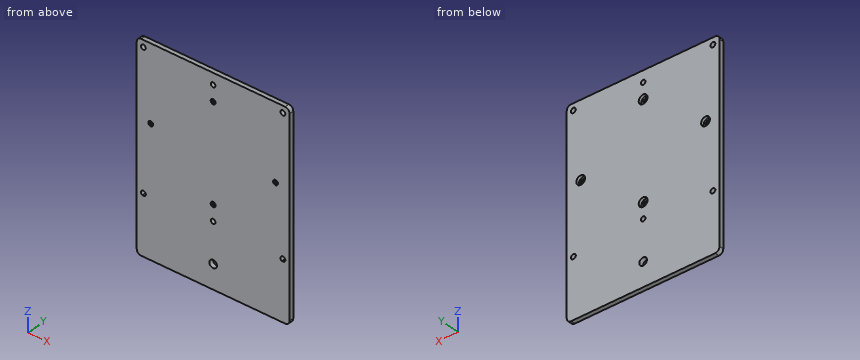
from build123d import *

# Parameters (mm, degrees)
SKETCH_1_W                   = 104
SKETCH_1_H                   = 100
EXTRUDE_1_DEPTH              = 3
HOLE_WIZARD_3_3_3_3_1_D      = 3.3
HOLE_WIZARD_M3_1_D           = 3.3
HOLE_WIZARD_M3_1_CBORE_D     = 6
HOLE_WIZARD_M3_1_CBORE_DEPTH = 2
FILLET_1_R                   = 3
SKETCH_49_R                  = 1.55
CUT_EXTRUDE_44_DEPTH         = 145.308696897
SKETCH_50_W                  = 104
SKETCH_50_H                  = 38
EXTRUDE_2_DEPTH              = 3
SKETCH_51_R                  = 2.6
CUT_EXTRUDE_45_DEPTH         = 145.308696897
FILLET_2_R                   = 3


with BuildPart() as part:
    # 草图1 → 凸台-拉伸1 (new body)
    with BuildSketch(Plane.XZ):
        with Locations((52, 50)):
            Rectangle(SKETCH_1_W, SKETCH_1_H)
    extrude(amount=-EXTRUDE_1_DEPTH)

    # Ø3.3 (3.3) 直径孔1 (through all)
    with Locations(Plane(origin=(0, 0, 0), x_dir=(-1, 0, 0), z_dir=(0, -1, 0))):
        with Locations((-4.5, -4.5), (-99.5, -4.5), (-99.5, -95.5), (-4.5, -95.5)):
            Hole(HOLE_WIZARD_3_3_3_3_1_D / 2)

    # M3 六角头机械螺钉的柱形沉头孔1 (through all)
    with Locations(Plane(origin=(0, 3, 0), x_dir=(1, 0, 0), z_dir=(0, 1, 0))):
        with Locations((52, -18), (94.5, -50), (9.5, -50), (52, -82)):
            CounterBoreHole(HOLE_WIZARD_M3_1_D / 2, HOLE_WIZARD_M3_1_CBORE_D / 2, HOLE_WIZARD_M3_1_CBORE_DEPTH)

    # 圆角1
    fillet_1_edges = [part.edges().sort_by_distance(p)[0] for p in [
        (0, 1.5, 100),
        (104, 1.5, 100),
        (104, 1.5, 0),
        (0, 1.5, 0),
    ]]
    fillet(fillet_1_edges, radius=FILLET_1_R)

    # 草图49 → 切除-拉伸44 (cut, through all)
    with BuildSketch(Plane(origin=(0, 3, 0), x_dir=(1, 0, 0), z_dir=(0, 1, 0))):
        with Locations(Location((52, -7.5, 0), (0, 0, 270))):
            Circle(SKETCH_49_R)
        with Locations(Location((52, -92.5, 0), (0, 0, 90))):
            Circle(SKETCH_49_R)
    extrude(amount=-CUT_EXTRUDE_44_DEPTH, mode=Mode.SUBTRACT)

    # 草图50 → 凸台-拉伸2 (add)
    with BuildSketch(Plane(origin=(0, 3, 0), x_dir=(1, 0, 0), z_dir=(0, 1, 0))):
        with Locations((52, 16)):
            Rectangle(SKETCH_50_W, SKETCH_50_H)
    extrude(amount=-EXTRUDE_2_DEPTH)

    # 草图51 → 切除-拉伸45 (cut, through all)
    with BuildSketch(Plane(origin=(0, 3, 0), x_dir=(1, 0, 0), z_dir=(0, 1, 0))):
        with Locations(Location((52, 19, 0), (0, 0, 270))):
            Circle(SKETCH_51_R)
    extrude(amount=-CUT_EXTRUDE_45_DEPTH, mode=Mode.SUBTRACT)

    # 圆角2
    fillet_2_edges = [part.edges().sort_by_distance(p)[0] for p in [
        (104, 1.5, -35),
        (0, 1.5, -35),
    ]]
    fillet(fillet_2_edges, radius=FILLET_2_R)


solid = part.part
Work out the finished part from the listing and answer in its coordinate system (mm). Give positions to 0.01 mm unless a question says otherwise; leave off trailing zeros. Order: outer loops, then holes, each group sorted by start corner. A loop starts at its lowest first (then second) coordinate and runs counter-clockwise, first axis right, second up. Notation, with made-up numbers: (11, 37) -> (59, 37) arc R31 ccw to (59, 73) -> close; hole circle Ø11 at (-33, 23). An arc over 180 degrees is marked (long way). One line per item, written item: value.
Item 1: Find section B-B, the plane z = -19. Give the vertices of the cut face in (x, y), plus the area to 3 significant figures.
Answer sheet:
outline: (0, 0) -> (49.4, 0) -> (49.4, 3) -> (0, 3) -> close; (54.6, 0) -> (104, 0) -> (104, 3) -> (54.6, 3) -> close
area: 296 mm²
Item 2: Straight lines are drawn through the part: probe 1 along X at (y, z) = (1.45, 50); probe 2 along Z at (x, y) = (99.5, 2.2); probe 3 along X at (y, z) = (2.3, 4.5). For each, find the intervals that lie inside material, in ascending order.
Answer sheet:
probe 1: 0 to 6.5, 12.5 to 91.5, 97.5 to 104
probe 2: -35 to 3, 6.15 to 93.85, 97.15 to 100
probe 3: 0 to 2.85, 6.15 to 97.85, 101.15 to 104
Item 3: Find section D-D, the plane z = 18. Give the vertices of the cut face in (x, y), plus the area to 3 significant figures.
Answer sheet:
outline: (0, 0) -> (50.35, 0) -> (50.35, 1) -> (49, 1) -> (49, 3) -> (0, 3) -> close; (53.65, 0) -> (104, 0) -> (104, 3) -> (55, 3) -> (55, 1) -> (53.65, 1) -> close
area: 297 mm²
Item 4: A flat-ended cylindrical pin translates along its axis: P1, Ø3, axis at x = 51.5, z = 81.5, coming from the +Y side. Find the tip coordinate at first contact, or state that the pin passes through.
Answer sheet:
P1: y = 1
Item 5: Find section A-A, the plane z = 50. Give the vertices of the cut face in (x, y).
Answer sheet:
outline: (0, 0) -> (7.85, 0) -> (7.85, 1) -> (6.5, 1) -> (6.5, 3) -> (0, 3) -> close; (11.15, 0) -> (92.85, 0) -> (92.85, 1) -> (91.5, 1) -> (91.5, 3) -> (12.5, 3) -> (12.5, 1) -> (11.15, 1) -> close; (96.15, 0) -> (104, 0) -> (104, 3) -> (97.5, 3) -> (97.5, 1) -> (96.15, 1) -> close
Item 6: Find section C-C, the plane z = 4.5. Give the vertices of the cut face in (x, y), plus the area to 3 significant figures.
Answer sheet:
outline: (0, 0) -> (2.85, 0) -> (2.85, 3) -> (0, 3) -> close; (6.15, 0) -> (97.85, 0) -> (97.85, 3) -> (6.15, 3) -> close; (101.15, 0) -> (104, 0) -> (104, 3) -> (101.15, 3) -> close
area: 292 mm²
